Geometry: final body of the model. Coordinates: model frame, mm. A direction names the side the tool comes from. Round coordinates to 2 decimals unless told otherwise and drop trailing zeros. Loops run counter-clockwise (first coordinate to the right, second up) from the corner with the lowest first, then second, coordinate; pieces in that order, holes last. Notation, with made-up numbers: (-14, -34.75) - (11, -34.75) arc R19 cw to (11, -28.75) - close; hole circle Ø3 at (35.5, -3.75). An arc over 180 degrees is marked (long way). Answer as CSV lines item,"result".
from build123d import *

# Parameters (mm, degrees)
F3_DEPTH      = 27.001
F3_DEPTH_BACK = 27.001
F5_DEPTH      = 27.0010001
F5_DEPTH_BACK = 27.0010001


with BuildPart() as f1:
    # F0 (on Front) → F1 (revolve)
    with BuildSketch(Plane.XZ):
        with BuildLine():
            Line((0, 0), (0, -2))
            Line((0, -2), (26.5, -2))
            ThreePointArc((26.5, -2), (26.8535533906, -1.8535533906), (27, -1.5))
            Line((27, -1.5), (27, 0))
            Line((27, 0), (25, 0))
            Line((25, 0), (25, 4.25))
            Line((25, 4.25), (25.6464466094, 4.8964466094))
            ThreePointArc((25.6464466094, 4.8964466094), (25.7928932188, 5.25), (25.6464466094, 5.6035533906))
            Line((25.6464466094, 5.6035533906), (25.1464466094, 6.1035533906))
            ThreePointArc((25.1464466094, 6.1035533906), (24.984234935, 6.2119397663), (24.7928932188, 6.25))
            Line((24.7928932188, 6.25), (23.5, 6.25))
            ThreePointArc((23.5, 6.25), (23.1464466094, 6.1035533906), (23, 5.75))
            Line((23, 5.75), (23, 2))
            ThreePointArc((23, 2), (22.4142135624, 0.5857864376), (21, 0))
            Line((21, 0), (0, 0))
        make_face()
    revolve(axis=Axis((0, 0, 12.0319147983), (0, 0, 1)))

    # F2 (on Front) → F3 (cut, two sides)
    with BuildSketch(Plane.XZ) as f3_sk:
        with BuildLine():
            Line((2, 20), (-2, 20))
            Line((-2, 20), (-2, 1.5))
            ThreePointArc((-2, 1.5), (-1.5606601718, 0.4393398282), (-0.5, 0))
            Line((-0.5, 0), (0.5, 0))
            ThreePointArc((0.5, 0), (1.5606601718, 0.4393398282), (2, 1.5))
            Line((2, 1.5), (2, 20))
        make_face()
    extrude(amount=F3_DEPTH, mode=Mode.SUBTRACT)
    extrude(f3_sk.sketch, amount=-F3_DEPTH_BACK, mode=Mode.SUBTRACT)

    # F4 (on Right) → F5 (cut, two sides)
    with BuildSketch(Plane.YZ) as f5_sk:
        with BuildLine():
            Line((2, 1.5), (2, 20))
            Line((2, 20), (-2, 20))
            Line((-2, 20), (-2, 1.5))
            ThreePointArc((-2, 1.5), (-1.5606601718, 0.4393398282), (-0.5, 0))
            Line((-0.5, 0), (0.5, 0))
            ThreePointArc((0.5, 0), (1.5606601718, 0.4393398282), (2, 1.5))
        make_face()
    extrude(amount=-F5_DEPTH, mode=Mode.SUBTRACT)
    extrude(f5_sk.sketch, amount=F5_DEPTH_BACK, mode=Mode.SUBTRACT)


solid = f1.part
(1) Material intervals for line 1 along Y through (x, z) = (10, -0.5); line 2 along Z through (x, y) = (-5, -2.5); line 3 along X through (y, z) = (-9, 4.25), sorted ascending.
Findings below:
line 1,"-25.08 to 25.08"
line 2,"-2 to 0"
line 3,"-23.32 to -21.17, 21.17 to 23.32"
(2) Draft query along X for faces 4 (the face through (-16.104, 16.422, 3.849)), 5 (the face through (17, -17, 6.25)), 6 (the face through (-17.866, -17.487, 2.155)), 7 (the face through (2, -24, 4)). Return one class per face: pulls with the +X half, pulls with the -X half, needs draft (parallel to the pull), parting line crosses it, or undercut.
Findings below:
face 4,"undercut"
face 5,"needs draft"
face 6,"pulls with the -X half"
face 7,"undercut"
(3) Pin query (flat end, axial travel): P1, Ø3, axis at x = 25, z = 4.5, coming from the -Y side; P2, Ø1, axis at y = -3, z = 1, coming from the -X side; P3, Ø4, axis at x = 12.5, z = 1, coming from the +Y side. Return the tip coordinate at first contact, or that it passes through.
Findings below:
P1,"y = -10.3"
P2,"x = -24.87"
P3,"y = 24.76"
(4) Section A-A (z = 3.5). Output: boundary loops of the cut face in (x, y).
Findings below:
outline,"(-24.92, -2) arc R25 ccw to (-2, -24.92) - (-2, -22.91) arc R23 cw to (-22.91, -2) - close; (-24.92, 2) - (-22.91, 2) arc R23 cw to (-2, 22.91) - (-2, 24.92) arc R25 ccw to start; (2, -24.92) arc R25 ccw to (24.92, -2) - (22.91, -2) arc R23 cw to (2, -22.91) - close; (2, 22.91) arc R23 cw to (22.91, 2) - (24.92, 2) arc R25 ccw to (2, 24.92) - close"
(5) Access query for faces 1 (the face through (23.411, 1.347, 0.262)), 2 (the face through (-2, 24, 4)), 3 (the face through (17.487, -17.866, 2.155)). Directions: +Z, -Z, +X, -X, +Y, -Y. A direction counts if a zero-diameter tool reaches every point of the face in a straight line with its end or side. Return the directions, or none.
Findings below:
face 1,"+Z, +X, -X"
face 2,"+Z, +Y, -Y"
face 3,"+X, -Y"
